from build123d import *

# Parameters (mm, degrees)
EXTRUDE_1_DEPTH          = 16
CUT_EXTRUDE_1_DEPTH      = 42.30909883
CUT_EXTRUDE_1_DEPTH_BACK = 42.30909883
SKETCH_4_R               = 3
CUT_EXTRUDE_2_DEPTH      = 23
CUT_EXTRUDE_3_DEPTH      = 42.30909883
CUT_EXTRUDE_3_DEPTH_BACK = 42.30909883
SKETCH_8_R               = 0.219313102
CUT_EXTRUDE_4_DEPTH      = 50.743759871


with BuildPart() as part:
    # 草图1 → 凸台-拉伸1 (new, symmetric)
    with BuildSketch(Plane(origin=(0, 0, 0), x_dir=(1, 0, 0), z_dir=(0, 1, 0))):
        Polygon((-14.5, 30), (14.5, 30), (23.461492837, 2.419361027), (0, -14.626411289), (-23.461492837, 2.419361027), align=None)
    extrude(amount=EXTRUDE_1_DEPTH, both=True)

    # 草图3 → 切除-拉伸1 (cut, two sides: drawn at the far end of the back side and taken through both)
    with BuildSketch(Plane(origin=(0, 0, 0), x_dir=(0, 0, -1), z_dir=(1, 0, 0)).offset(-CUT_EXTRUDE_1_DEPTH_BACK)):
        Polygon((6, 16), (6, 8), (30, -8), (30, 16), align=None)
    extrude(amount=CUT_EXTRUDE_1_DEPTH + CUT_EXTRUDE_1_DEPTH_BACK, mode=Mode.SUBTRACT)

    # 草图4 → 切除-拉伸2 (cut)
    with BuildSketch(Plane(origin=(21.932151994, 0, -7.126188163), x_dir=(-0.3090169943749527, 0, -0.9510565162951519), z_dir=(0.951056516295152, 0, -0.3090169943749527))):
        with Locations((14.05094907, -11)):
            Circle(SKETCH_4_R)
    cut_extrude_2 = extrude(amount=-CUT_EXTRUDE_2_DEPTH, mode=Mode.SUBTRACT)

    # 镜向1: 切除-拉伸2 across plane
    add(cut_extrude_2.mirror(Plane(origin=(0, 0, 0), x_dir=(0, 0, 1), z_dir=(1, 0, 0))), mode=Mode.SUBTRACT)

    # 草图7 → 切除-拉伸3 (cut, two sides: drawn at the far end of the back side and taken through both)
    with BuildSketch(Plane.XY.offset(-CUT_EXTRUDE_3_DEPTH_BACK)):
        Polygon((0, 8), (-1.909830056, 2.122147477), (-8.090169944, 2.122147477), (-3.090169944, -1.510565163), (-5, -7.388417686), (0, -3.755705046), (5, -7.388417686), (3.090169944, -1.510565163), (8.090169944, 2.122147477), (1.909830056, 2.122147477), align=None)
    extrude(amount=CUT_EXTRUDE_3_DEPTH + CUT_EXTRUDE_3_DEPTH_BACK, mode=Mode.SUBTRACT)

    # 草图8 → 切除-拉伸4 (cut, through all)
    with BuildSketch(Plane(origin=(0, 16, 0), x_dir=(1, 0, 0), z_dir=(0, 1, 0))):
        with Locations(Location((-0.775935465, 0.431354415, 0), (0, 0, 270))):
            Circle(SKETCH_8_R)
        with BuildLine():
            Line((-5.113847326, 2.420614591), (-5.113847326, 0))
            ThreePointArc((-5.113847326, 0), (-4.281010431, 0.832836895), (-3.448173537, 0))
            Line((-3.448173537, 0), (-3.448173537, -2.420614591))
            ThreePointArc((-3.448173537, -2.420614591), (-3.698173537, -2.670614591), (-3.948173537, -2.420614591))
            Line((-3.948173537, -2.420614591), (-3.948173537, -0.536873711))
            ThreePointArc((-3.948173537, -0.536873711), (-4.531010431, 0.045963183), (-5.113847326, -0.536873711))
            Line((-5.113847326, -0.536873711), (-5.113847326, -2.420614591))
            ThreePointArc((-5.113847326, -2.420614591), (-5.363847326, -2.670614591), (-5.613847326, -2.420614591))
            Line((-5.613847326, -2.420614591), (-5.613847326, 2.420614591))
            ThreePointArc((-5.613847326, 2.420614591), (-5.363847326, 2.670614591), (-5.113847326, 2.420614591))
        make_face()
        with BuildLine():
            Line((-1.013410033, 0), (-1.013410033, -2.420614591))
            ThreePointArc((-1.013410033, -2.420614591), (-0.775935465, -2.658089159), (-0.538460898, -2.420614591))
            Line((-0.538460898, -2.420614591), (-0.538460898, 0))
            Line((-0.538460898, 0), (-1.013410033, 0))
        make_face()
        with BuildLine():
            Line((2.187750175, 0), (2.187750175, -2.420614591))
            Line((2.187750175, -2.420614591), (2.64847422, -2.420614591))
            Line((2.64847422, -2.420614591), (2.64847422, -0.984785713))
            ThreePointArc((2.64847422, -0.984785713), (2.926986903, -0.70627303), (3.205499587, -0.984785713))
            Line((3.205499587, -0.984785713), (3.205499587, -2.420614591))
            Line((3.205499587, -2.420614591), (3.610975114, -2.420614591))
            Line((3.610975114, -2.420614591), (3.610975114, -0.622613397))
            ThreePointArc((3.610975114, -0.622613397), (3.129724667, -0.14136295), (2.64847422, -0.622613397))
            Line((2.64847422, -0.622613397), (2.64847422, 0))
            Line((2.64847422, 0), (2.187750175, 0))
        make_face()
        with BuildLine():
            ThreePointArc((-8.375, 2.420614591), (-11.5, 0), (-8.375, -2.420614591))
            ThreePointArc((-8.375, -2.420614591), (-8.015877082, -1.811491673), (-8.625, -1.452368755))
            ThreePointArc((-8.625, -1.452368755), (-10.5, 0), (-8.625, 1.452368755))
            ThreePointArc((-8.625, 1.452368755), (-8.015877082, 1.811491673), (-8.375, 2.420614591))
        make_face()
        with BuildLine():
            ThreePointArc((9.512511285, -1.753375111), (7.583787314, -0.99482991), (9.364950424, -2.05446426))
            ThreePointArc((9.364950424, -2.05446426), (9.507618037, -2.354597316), (9.820725394, -2.465942199))
            ThreePointArc((9.820725394, -2.465942199), (9.943547456, -2.381589693), (9.923856182, -2.233897927))
            ThreePointArc((9.923856182, -2.233897927), (9.6186642, -2.078828836), (9.512511285, -1.753375111))
        make_face()
    extrude(amount=-CUT_EXTRUDE_4_DEPTH, mode=Mode.SUBTRACT)


solid = part.part
The listing builds one solid part. Answer for the finished solid, in the listing's coordinates (mm). A direction names the side the tool comes from. Round coordinates to 2 decimals unless told otherwise and drop trailing zeros. Write each loop counter-clockwise with the first axis right and the second up, starting at its lowest first coordinate (ties: lowest second). Pieces come first, ordered by that corner, then holes. Notation, with made-up numbers: M 78,4 L 88,4 A33 cw 88,41 Z; hole C -7.5,65.25 d11. An arc over 180 degrees is marked long. Write each question's results on one line, items separated by ' | '. Start each with the question number.
Item 1: Which of the six approach directions +Z, -Z, +X, -X, +Y, -Y give full straight-line access (tool end or side, diameter ignored) to faces 3 (the flat face through (-4.037, -10.958, -12.622)), 4 (the flat face through (3.205, -11, 2))?
Item 2: Find section C-C on z = 6. Write down the section's boundary in (x, y), and give its area (3 significant figures).
Item 3: Find section A-A on y = 7. Give the number of separate pieces and of enclosed holes in the cut face, and give its area (3 significant figures).
Item 4: Straight lines are drawn through the part: probe 1 along X at (y, z) = (-4.5, 10.5); probe 2 along Z at (x, y) = (8, -9); probe 3 along Z at (x, y) = (-9, 0). For each, find the intervals that lie inside material, in ascending order.
Item 5: Find section D-D on x = 20.5. Write down the section's boundary in (y, z).
Item 6: Given pin 1 Ø1.6 at (y, z) = (-12, 1.5) entering from +X; pin 2 Ø0.7 at (y, z) = (13.5, 1.5) entering from -X; pin 3 Ø2.5 at (y, z) = (6, 1.5) entering from +X, each flat-ended and moving along its own axis, determine where each tip first touches the part or whether it passes through.
Item 7: The mould has two halves that part along X. Classify faces 1 (the cylindrical face through (1.66, -10.91, -11.08)), 2 (the flat face through (0, 12, -6)): +X half, -X half, draft (parallel to the pull), parting line (faces both ways), or undercut.
Answer block:
1) face 3: none | face 4: +Y, -Y
2) outline: M -11.87,-16 L 11.87,-16 L 11.87,16 L -11.87,16 Z; hole M -8.09,2.12 L -3.09,-1.51 L -5,-7.39 L 0,-3.76 L 5,-7.39 L 3.09,-1.51 L 8.09,2.12 L 1.91,2.12 L 0,8 L -1.91,2.12 Z | area: 679 mm²
3) separate pieces: 2 | enclosed holes: 6 | area: 595 mm²
4) probe 1: x = -5.68 to -4.06, -1.02 to 1.02, 4.06 to 5.68 | probe 2: z = -30 to -19.72, -15.02 to 0.55, 2.35 to 8.81 | probe 3: z = -18 to -2.5, -1.5 to 1.5, 2.5 to 8.09
5) outline: M -16,-11.53 L 4.31,-11.53 L 8,-6 L 16,-6 L 16,-0.27 L -16,-0.27 Z
6) pin 1: stops at x = 19.17 | pin 2: stops at x = -18.55 | pin 3: stops at x = 19.79
7) face 1: undercut | face 2: draft
